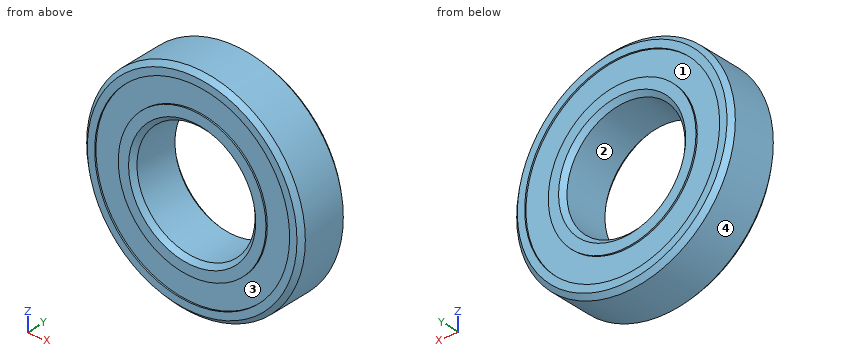
```python
from build123d import *

# Parameters (mm, degrees)
F0_R     = 18.5
F0_R_2   = 10
F1_DEPTH = 9
F2_SIZE  = 0.762
F3_R     = 16.5
F3_R_2   = 12.5
F4_DEPTH = 0.254
F5_R     = 16.5
F5_R_2   = 12.5
F6_DEPTH = 0.254


with BuildPart() as f1:
    # F0 (on Front) → F1 (new body)
    with BuildSketch(Plane.XZ):
        Circle(F0_R)
        Circle(F0_R_2, mode=Mode.SUBTRACT)
    extrude(amount=F1_DEPTH)

    # F2
    f2_edges = [f1.edges().sort_by_distance(p)[0] for p in [
        (18.5, -4.5, 0),
        (-18.5, 0, 0),
        (-18.5, -9, 0),
        (10, -4.5, 0),
        (-10, 0, 0),
        (-10, -9, 0),
    ]]
    chamfer(f2_edges, length=F2_SIZE)

    # F3 (on face) → F4 (cut)
    with BuildSketch(Plane(origin=(0, 0, 0), x_dir=(-1, 0, 0), z_dir=(0, 1, 0))):
        Circle(F3_R)
        Circle(F3_R_2, mode=Mode.SUBTRACT)
    extrude(amount=-F4_DEPTH, mode=Mode.SUBTRACT)

    # F5 (on face) → F6 (cut)
    with BuildSketch(Plane.XZ.offset(9)):
        Circle(F5_R)
        Circle(F5_R_2, mode=Mode.SUBTRACT)
    extrude(amount=-F6_DEPTH, mode=Mode.SUBTRACT)


solid = f1.part
```
Can you work these out from the model? Positions are in its coordinate system, mm. Face numbers are marked on the shaded views. A direction names the side the tool comes from. Coordinates: 2 decimals unless noted, no trailing zeros. Loops run counter-clockwise (first coordinate to the right, second up) from the corner with the lowest first, then second, coordinate; pieces in that order, holes last. Notation, with made-up numbers: M -7.5,85.25 L 6.5,85.25 A24 cw 6.5,113.25 Z; hole C 63.25,56 d11. An arc over 180 degrees is marked long. Put each result on its own line as item: value. Start each with the question number.
(1) I need wall thicknesses on probe 1 along Z at (x, y) = (0, -3); probe 2 along Z at (x, y) = (0, -8.85); probe 3 along Z at (x, y) = (0, -8.9). Which ranges of each line are inside material? Lowest first, please.
(2) We'd pull the mould along Z, two halves only. Please class the marked faces 3 and 4: +Z half, -Z half, draft (parallel to the pull), parting line (faces both ways), or undercut.
(3) Will these pins go through, and if not, where does the flat tip stop? pin 1 Ø5 at (x, y) = (-4.5, -7.5) entering from +Z; pin 2 Ø12 at (x, z) = (0.5, -2.5) entering from +Y; pin 3 Ø5 at (x, y) = (-13, -4.5) entering from +Z; pin 4 Ø3 at (x, y) = (13, -5.5) entering from +Z.
(4) Which directions (+Z, -Z, +X, -X, +Y, -Y) give clear straight access to the entire face, cutting with the end or side of a thin tool? Please do the marked faces 1 and 2.
(5) Imagine slicing it at C-C on y = -4. List the corners of the cut face in (x, z) for me.
Worked answers:
1. probe 1: z = -18.5 to -10, 10 to 18.5
1. probe 2: z = -17.89 to -16.5, -12.5 to -10.61, 10.61 to 12.5, 16.5 to 17.89
1. probe 3: z = -17.84 to -16.5, -12.5 to -10.66, 10.66 to 12.5, 16.5 to 17.84
2. face 3: undercut
2. face 4: parting line
3. pin 1: stops at z = 18.39
3. pin 2: passes through
3. pin 3: stops at z = 15.23
3. pin 4: stops at z = 14.49
4. face 1: +Y
4. face 2: +Y, -Y
5. outline: C 0,0 d37; hole C 0,0 d20
